```python
from build123d import *

# Parameters (mm, degrees)
BOSS_EXTRUDE1_DEPTH = 0.5


with BuildPart() as part:
    # Model → Boss-Extrude1 (new body)
    with BuildSketch(Plane.XY):
        with BuildLine():
            Line((1561.604350415, 393.6), (1562.977857238, 393.6))
            ThreePointArc((1562.977857238, 393.6), (1563.227857238, 393.533012702), (1563.41086994, 393.35))
            Line((1563.41086994, 393.35), (1566.644031447, 387.75))
            ThreePointArc((1566.644031447, 387.75), (1566.827044149, 387.566987298), (1567.077044149, 387.5))
            Line((1567.077044149, 387.5), (1568.831847468, 387.5))
            ThreePointArc((1568.831847468, 387.5), (1569.118635686, 387.590423978), (1569.301693779, 387.828989928))
            Line((1569.301693779, 387.828989928), (1572.556322945, 396.771010072))
            ThreePointArc((1572.556322945, 396.771010072), (1572.739381037, 397.009576022), (1573.026169255, 397.1))
            Line((1573.026169255, 397.1), (1574.399676079, 397.1))
            ThreePointArc((1574.399676079, 397.1), (1574.649676079, 397.033012702), (1574.83268878, 396.85))
            Line((1574.83268878, 396.85), (1578.643200557, 390.25))
            ThreePointArc((1578.643200557, 390.25), (1578.826213259, 390.066987298), (1579.076213259, 390))
            Line((1579.076213259, 390), (1581.687538124, 390))
            ThreePointArc((1581.687538124, 390), (1582.041091515, 390.146446609), (1582.187538124, 390.5))
            Line((1582.187538124, 390.5), (1582.187538124, 409.5))
            ThreePointArc((1582.187538124, 409.5), (1582.041091515, 409.853553391), (1581.687538124, 410))
            Line((1581.687538124, 410), (1579.076213259, 410))
            ThreePointArc((1579.076213259, 410), (1578.826213259, 409.933012702), (1578.643200557, 409.75))
            Line((1578.643200557, 409.75), (1574.83268878, 403.15))
            ThreePointArc((1574.83268878, 403.15), (1574.649676079, 402.966987298), (1574.399676079, 402.9))
            Line((1574.399676079, 402.9), (1573.026169255, 402.9))
            ThreePointArc((1573.026169255, 402.9), (1572.739381037, 402.990423978), (1572.556322945, 403.228989928))
            Line((1572.556322945, 403.228989928), (1569.301693779, 412.171010072))
            ThreePointArc((1569.301693779, 412.171010072), (1569.118635686, 412.409576022), (1568.831847468, 412.5))
            Line((1568.831847468, 412.5), (1567.077044149, 412.5))
            ThreePointArc((1567.077044149, 412.5), (1566.827044149, 412.433012702), (1566.644031447, 412.25))
            Line((1566.644031447, 412.25), (1563.41086994, 406.65))
            ThreePointArc((1563.41086994, 406.65), (1563.227857238, 406.466987298), (1562.977857238, 406.4))
            Line((1562.977857238, 406.4), (1561.604350415, 406.4))
            ThreePointArc((1561.604350415, 406.4), (1561.317562197, 406.490423978), (1561.134504104, 406.728989928))
            Line((1561.134504104, 406.728989928), (1558.243845172, 414.671010072))
            ThreePointArc((1558.243845172, 414.671010072), (1558.06078708, 414.909576022), (1557.773998862, 415))
            Line((1557.773998862, 415), (1556.019195543, 415))
            ThreePointArc((1556.019195543, 415), (1555.769195543, 414.933012702), (1555.586182841, 414.75))
            Line((1555.586182841, 414.75), (1553.132444197, 410.5))
            ThreePointArc((1553.132444197, 410.5), (1552.766418793, 410.133974596), (1552.266418793, 410))
            Line((1552.266418793, 410), (1544.072525617, 410))
            ThreePointArc((1544.072525617, 410), (1530.843769062, 405), (1517.615012507, 410))
            Line((1517.615012507, 410), (1509.421119331, 410))
            ThreePointArc((1509.421119331, 410), (1508.921119331, 410.133974596), (1508.555093928, 410.5))
            Line((1508.555093928, 410.5), (1506.101355284, 414.75))
            ThreePointArc((1506.101355284, 414.75), (1505.918342582, 414.933012702), (1505.668342582, 415))
            Line((1505.668342582, 415), (1503.913539263, 415))
            ThreePointArc((1503.913539263, 415), (1503.626751044, 414.909576022), (1503.443692952, 414.671010072))
            Line((1503.443692952, 414.671010072), (1500.55303402, 406.728989928))
            ThreePointArc((1500.55303402, 406.728989928), (1500.369975928, 406.490423978), (1500.08318771, 406.4))
            Line((1500.08318771, 406.4), (1498.709680887, 406.4))
            ThreePointArc((1498.709680887, 406.4), (1498.459680886, 406.466987298), (1498.276668185, 406.65))
            Line((1498.276668185, 406.65), (1495.043506677, 412.25))
            ThreePointArc((1495.043506677, 412.25), (1494.860493975, 412.433012702), (1494.610493975, 412.5))
            Line((1494.610493975, 412.5), (1492.855690656, 412.5))
            ThreePointArc((1492.855690656, 412.5), (1492.568902438, 412.409576022), (1492.385844346, 412.171010072))
            Line((1492.385844346, 412.171010072), (1489.131215179, 403.228989928))
            ThreePointArc((1489.131215179, 403.228989928), (1488.948157087, 402.990423978), (1488.661368869, 402.9))
            Line((1488.661368869, 402.9), (1487.287862046, 402.9))
            ThreePointArc((1487.287862046, 402.9), (1487.037862046, 402.966987298), (1486.854849344, 403.15))
            Line((1486.854849344, 403.15), (1483.044337567, 409.75))
            ThreePointArc((1483.044337567, 409.75), (1482.861324865, 409.933012702), (1482.611324865, 410))
            Line((1482.611324865, 410), (1480, 410))
            ThreePointArc((1480, 410), (1479.646446609, 409.853553391), (1479.5, 409.5))
            Line((1479.5, 409.5), (1479.5, 390.5))
            ThreePointArc((1479.5, 390.5), (1479.646446609, 390.146446609), (1480, 390))
            Line((1480, 390), (1482.611324865, 390))
            ThreePointArc((1482.611324865, 390), (1482.861324865, 390.066987298), (1483.044337567, 390.25))
            Line((1483.044337567, 390.25), (1486.854849344, 396.85))
            ThreePointArc((1486.854849344, 396.85), (1487.037862046, 397.033012702), (1487.287862046, 397.1))
            Line((1487.287862046, 397.1), (1488.661368869, 397.1))
            ThreePointArc((1488.661368869, 397.1), (1488.948157087, 397.009576022), (1489.131215179, 396.771010072))
            Line((1489.131215179, 396.771010072), (1492.385844346, 387.828989928))
            ThreePointArc((1492.385844346, 387.828989928), (1492.568902438, 387.590423978), (1492.855690656, 387.5))
            Line((1492.855690656, 387.5), (1494.610493975, 387.5))
            ThreePointArc((1494.610493975, 387.5), (1494.860493975, 387.566987298), (1495.043506677, 387.75))
            Line((1495.043506677, 387.75), (1498.276668185, 393.35))
            ThreePointArc((1498.276668185, 393.35), (1498.459680886, 393.533012702), (1498.709680887, 393.6))
            Line((1498.709680887, 393.6), (1500.08318771, 393.6))
            ThreePointArc((1500.08318771, 393.6), (1500.369975928, 393.509576022), (1500.55303402, 393.271010072))
            Line((1500.55303402, 393.271010072), (1503.443692952, 385.328989928))
            ThreePointArc((1503.443692952, 385.328989928), (1503.626751044, 385.090423978), (1503.913539263, 385))
            Line((1503.913539263, 385), (1505.668342582, 385))
            ThreePointArc((1505.668342582, 385), (1505.918342582, 385.066987298), (1506.101355283, 385.25))
            Line((1506.101355283, 385.25), (1508.555093928, 389.5))
            ThreePointArc((1508.555093928, 389.5), (1508.921119331, 389.866025404), (1509.421119331, 390))
            Line((1509.421119331, 390), (1517.615012507, 390))
            ThreePointArc((1517.615012507, 390), (1530.843769062, 395), (1544.072525618, 390))
            Line((1544.072525618, 390), (1552.266418793, 390))
            ThreePointArc((1552.266418793, 390), (1552.766418793, 389.866025404), (1553.132444197, 389.5))
            Line((1553.132444197, 389.5), (1555.586182841, 385.25))
            ThreePointArc((1555.586182841, 385.25), (1555.769195543, 385.066987298), (1556.019195543, 385))
            Line((1556.019195543, 385), (1557.773998862, 385))
            ThreePointArc((1557.773998862, 385), (1558.06078708, 385.090423978), (1558.243845172, 385.328989928))
            Line((1558.243845172, 385.328989928), (1561.134504104, 393.271010072))
            ThreePointArc((1561.134504104, 393.271010072), (1561.317562197, 393.509576022), (1561.604350415, 393.6))
        make_face()
    extrude(amount=BOSS_EXTRUDE1_DEPTH)


solid = part.part
```
For this review, take the finished solid that the model builds, in its own axes (mm). A direction names the side the tool comes from. Round coordinates to 2 decimals unless told otherwise and drop trailing zeros. Write each loop counter-clockwise with the first axis right and the second up, starting at its lowest first coordinate (ties: lowest second). Pieces come first, ordered by that corner, then holes. Notation, with made-up numbers: (82.5, 37.5) -> (109.5, 37.5) arc R12 cw to (109.5, 55.5) -> close; hole circle Ø4 at (-35.75, 35). An arc over 180 degrees is marked (long way). Use one line per item in the form item = value.
1) Take a section at A-A, the plane x = 1559.5. Write out the cut boundary in (y, z).
Found:
outline = (388.78, 0) -> (411.22, 0) -> (411.22, 0.5) -> (388.78, 0.5) -> close
2) To check wall thickness, follow L1, parallel to X at y = 389, z = 0.45; L2, parallel to X at y = 407, z = 0.4; L3, parallel to X at y = 388.5, z = 0.1. State the ranges of each line that lie inside material, in increasing order. Write a range as from..to.
Found:
L1 = 1491.96..1495.77, 1502.11..1508.27, 1553.42..1559.58, 1565.92..1569.73
L2 = 1479.5..1484.63, 1490.5..1498.07, 1500.65..1522.13, 1539.56..1561.04, 1563.61..1571.18, 1577.06..1582.19
L3 = 1492.14..1495.48, 1502.29..1507.98, 1553.71..1559.4, 1566.21..1569.55
3) Mouldability with a two-part tool opening along X and no side actions: class faces 1 (the flat face through (1530, 400, 0)), 2 (the flat face through (1570.95, 407.64, 0.25)) as +X half, -X half, draft (parallel to the pull), parting line (faces both ways), or undercut.
Found:
face_1 = draft
face_2 = undercut
4) Tool access review of faces 3 (the flat face through (1554.342, 387.405, 0.246)), 4 (the flat face through (1507.345, 412.595, 0.246)): name each direction out of +Z, -Z, +X, -X, +Y, -Y from which nothing blocks a thin tool from reaching the whole face with its end or side.
Found:
face_3 = +Z, -Z, -Y
face_4 = +Z, -Z, +Y
5) Take a section at B-B, the plane x = 1520.5. Write out the cut boundary in (y, z), and give its area (3 significant figures).
Found:
outline = (392.12, 0) -> (407.88, 0) -> (407.88, 0.5) -> (392.12, 0.5) -> close
area = 7.88 mm2
